Can you work these out from the model? Positions are in its coordinate system, mm. A direction names the side the tool comes from. Coordinates: 2 decimals unless noted, no trailing zeros. Order: outer loops, then holes, each group sorted by start corner. A loop starts at its lowest first (then second) coordinate and runs counter-clockwise, first axis right, second up.
```python
from build123d import *

# Parameters (mm, degrees)
SKETCH1_R           = 35.3139375
BOSS_EXTRUDE1_DEPTH = 6.35


with BuildPart() as part:
    # Sketch1 → Boss-Extrude1 (new body)
    with BuildSketch(Plane.XY):
        Polygon((36.4109, 35.3139375), (30.0609, 35.3139375), (30.0609, 41.6639375), (-28.9639375, 41.6639375), (-28.9639375, 35.3139375), (-35.3139375, 35.3139375), (-35.3139375, 28.9639375), (-41.6639375, 28.9639375), (-41.6639375, -28.9639375), (-35.3139375, -28.9639375), (-35.3139375, -35.3139375), (-28.9639375, -35.3139375), (-28.9639375, -41.6639375), (30.0609, -41.6639375), (30.0609, -35.3139375), (36.4109, -35.3139375), (36.4109, -28.9639375), (42.7609, -28.9639375), (42.7609, 28.9639375), (36.4109, 28.9639375), align=None)
        Circle(SKETCH1_R, mode=Mode.SUBTRACT)
    extrude(amount=-BOSS_EXTRUDE1_DEPTH)


solid = part.part
```
1. Imagine slicing it at A-A on z = -3. Please give me the cut outline in (x, y), then the cut area to 3 significant figures.
Completed:
outline: (-41.66, -28.96) - (-35.31, -28.96) - (-35.31, -35.31) - (-28.96, -35.31) - (-28.96, -41.66) - (30.06, -41.66) - (30.06, -35.31) - (36.41, -35.31) - (36.41, -28.96) - (42.76, -28.96) - (42.76, 28.96) - (36.41, 28.96) - (36.41, 35.31) - (30.06, 35.31) - (30.06, 41.66) - (-28.96, 41.66) - (-28.96, 35.31) - (-35.31, 35.31) - (-35.31, 28.96) - (-41.66, 28.96) - close; hole circle Ø70.63 at (0, 0)
area: 2,630 mm2
2. Imagine slicing it at B-B on x = 0. Please give me the cut outline in (y, z).
Completed:
outline: (-41.66, -6.35) - (-35.31, -6.35) - (-35.31, 0) - (-41.66, 0) - close; (35.31, -6.35) - (41.66, -6.35) - (41.66, 0) - (35.31, 0) - close
3. Please list where these lines run through material, in increasing order: probe 1 along Y at (x, z) = (0, -3.5); probe 2 along X at (y, z) = (37, -0.25); probe 3 along Y at (x, z) = (-7, -0.25).
Completed:
probe 1: y = -41.66 to -35.31, 35.31 to 41.66
probe 2: x = -28.96 to 30.06
probe 3: y = -41.66 to -34.61, 34.61 to 41.66
4. I'm going to push flat-ended pins straight in: pin 1 (1.9 mm diameter, centred on y = -37.5, z = -2.5, fed in from -X); pin 2 (3 mm diameter, centred on x = -32, z = -2, fed in from +Y); pin 3 (2 mm diameter, centred on y = -30.5, z = -3, fed in from -X). Where does each tip first touch, or does it pass through?
Completed:
pin 1: stops at x = -28.96
pin 2: stops at y = 35.31
pin 3: stops at x = -35.31
5. Imagine slicing it at C-C on y = -24. Please give me the cut outline in (x, z), then the cut area to 3 significant figures.
Completed:
outline: (-41.66, -6.35) - (-25.91, -6.35) - (-25.91, 0) - (-41.66, 0) - close; (25.91, -6.35) - (42.76, -6.35) - (42.76, 0) - (25.91, 0) - close
area: 207 mm2
6. Imagine slicing it at D-D on x = -36.5. Please give me the cut outline in (y, z).
Completed:
outline: (-28.96, -6.35) - (28.96, -6.35) - (28.96, 0) - (-28.96, 0) - close
7. On a 3-axis mill with a long thin cutter (end or side, diameter ignored), from which of +Z, -Z, +X, -X, +Y, -Y can I reach the whole of each face in a straight line? I mean faces 1 (the flat face through (40, 28.964, -3)), 2 (the flat face through (-28.964, -38, -3)), 3 (the flat face through (-28.964, 39, -3)), 4 (the flat face through (40, -28.964, -3)). Say none if no direction works.
Completed:
face 1: +Z, -Z, +X, +Y
face 2: +Z, -Z, -X, -Y
face 3: +Z, -Z, -X, +Y
face 4: +Z, -Z, +X, -Y
